Geometry: see drawing. Coordinates: mm, zero at the bounding-box minimum. A direction names the side the tool comes from. Coordinates: 2 decimals unless noted, no trailing zeros. Loops run counter-clockwise (first coordinate to the right, second up) from the corner with the lowest first, then second, coordinate; pieces in that order, holes last.
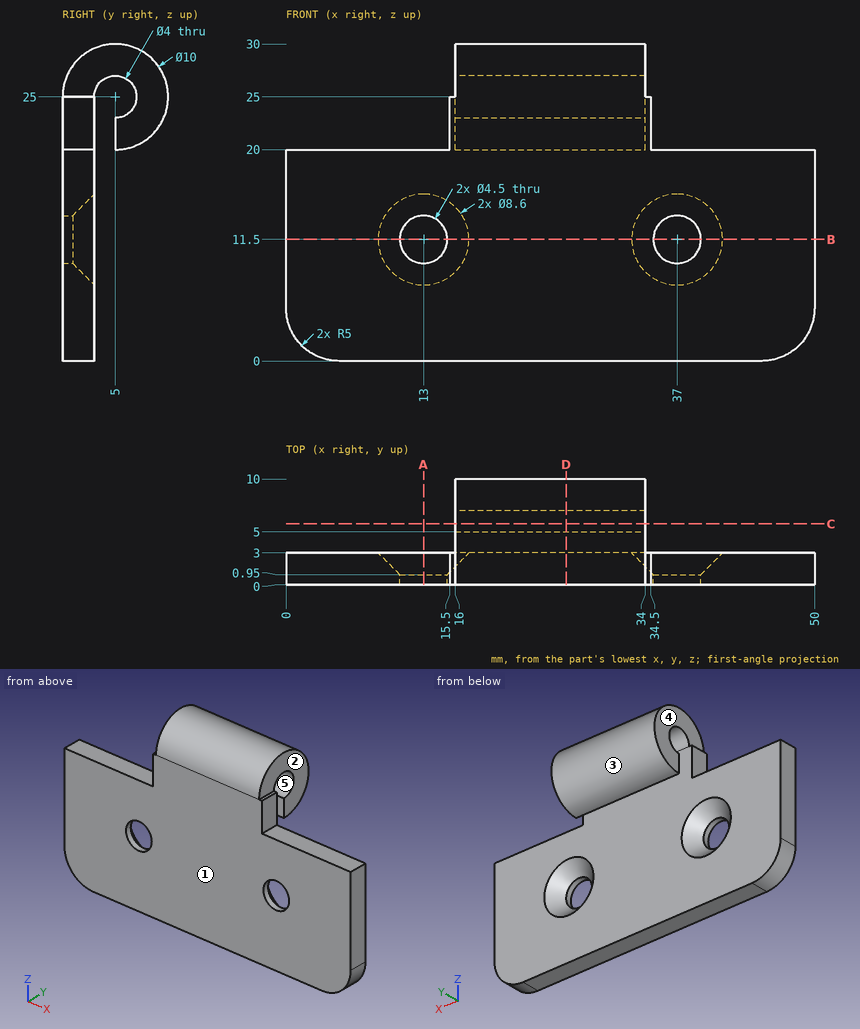
Item 1: Section query D-D (x = 26.5). Output: boundary loops of the cut face in (y, z), then the cut area to 3 significant figures.
Result:
outline: (0, 0) - (3, 0) - (3, 25) arc R2 cw (long way) to (5, 23) - (5, 20) arc R5 ccw (long way) to (0, 25) - close
area: 124 mm2
Item 2: Line query: L1, parallel to X at y = 0.45, z = 11.5; L2, parallel to Z at x = 37, y = 0.4; L3, parallel to Y at x = 24, z = 25. Output: solid intervals per line, ascending.
Result:
L1: x = 0 to 10.75, 15.25 to 34.75, 39.25 to 50
L2: z = 0 to 9.25, 13.75 to 20
L3: y = 0 to 3, 7 to 10
Item 3: Section query A-A (x = 13). Output: boundary loops of the cut face in (y, z), then the cut area to 3 significant figures.
Result:
outline: (0, 0) - (3, 0) - (3, 7.2) - (0.95, 9.25) - (0, 9.25) - close; (0, 13.75) - (0.95, 13.75) - (3, 15.8) - (3, 20) - (0, 20) - close
area: 42.3 mm2
Item 4: Contact query for flat-ended pins moving along their axis: P1, Ø5, axis at y = 4, z = 23, coming from the +X side; P2, Ø1.5, axis at x = 41, y = 1, coming from the +Z side; P3, Ø1.5, axis at y = 1.5, z = 22, coming from the -X side; P4, Ø4, axis at x = 37, z = 11.5, coming from the +Y side. Output: stop coordinate, or through.
Result:
P1: stops at x = 34.5
P2: stops at z = 20
P3: stops at x = 15.5
P4: passes through
Item 5: Section query B-B (z = 11.5). Output: boundary loops of the cut face in (x, y).
Result:
outline: (0, 0) - (10.75, 0) - (10.75, 0.95) - (8.7, 3) - (0, 3) - close; (15.25, 0) - (34.75, 0) - (34.75, 0.95) - (32.7, 3) - (17.3, 3) - (15.25, 0.95) - close; (39.25, 0) - (50, 0) - (50, 3) - (41.3, 3) - (39.25, 0.95) - close
Item 6: Reachability of the marked faces 1 and 2 from +Z, -Z, +X, -X, +Y, -Y: full face, straight path, thin tool, end or side. Return the list, or none.
Result:
face 1: +Z, -Z, +X, -X, -Y
face 2: +Z, +X, +Y
Item 7: Mould query, pull axis Z, two halves, no side actions, for the marked faces 3, 4 and 5. Classes: +Z half, -Z half, draft (parallel to the pull), parting line (faces both ways), or undercut.
Result:
face 3: parting line
face 4: draft
face 5: undercut
Item 8: Section query C-C (y = 5.75). Output: boundary loops of the cut face in (x, z), then the cut area to 3 significant figures.
Result:
outline: (16, 20.06) - (34, 20.06) - (34, 23.15) - (16, 23.15) - close; (16, 26.85) - (34, 26.85) - (34, 29.94) - (16, 29.94) - close
area: 111 mm2
